Answer from the drawing. Dimensions are ordinates in mm from the lowest x, y and z of the part. Round coordinates to 2 decimals unless told otherwise and drop trailing zeros. Order: outer loops, then holes, each group sorted by start corner. A loop starts at its lowest first (then second) coordinate and runs counter-clockwise, first axis right, second up. Notation, with made-up numbers: (12.25, 57) -> (69.25, 57) arc R27 cw to (69.25, 84) -> close; hole circle Ø11 at (56, 51.25). An arc over 180 degrees is marked (long way). Use a Markdown table: item, result. Add a question column.
1. Section A-A, the plane y = 2.5 is taken. Give the vertices of the cut face in (x, z) (1 decimal).
2. Consider L1, parallel to X at y = 5, z = 6.5 (1 decimal); L2, parallel to X at y = 4.5, z = 4.75 (1 decimal); L3, parallel to Z at x = 18, y = 5 (1 decimal). Determine where each line is inside the solid, lowest interval first. Write a range as [from, to].
3. Section B-B, the plane x = 7.5 is taken. Give the vertices of the cut face in (y, z) (1 decimal).
4. Given pin 1 (6 mm diameter, centred on x = 36.5, z = 4, fed in from +Y); pin 2 (1.5 mm diameter, centred on y = 6, z = 8, fed in from -X); pin 3 (1.5 mm diameter, centred on x = 9.5, z = 10, fed in from -Y); pin 4 (1 mm diameter, centred on y = 3.5, z = 10, fed in from +X), each flat-ended and moving along its own axis, determine where each tip first touches the part or whether it passes through.
5. Section C-C, the plane z = 8.75 is taken. Give the vertices of the cut face in (x, y) (1 decimal), then the cut area to 3 significant figures.
6. The mould has two halves that part along Y. Classify the marked faces 1, 2 and 3: +Y half, -Y half, draft (parallel to the pull), parting line (faces both ways), or undercut.
7. Section D-D, the plane x = 29.5 is taken. Give the vertices of the cut face in (y, z).
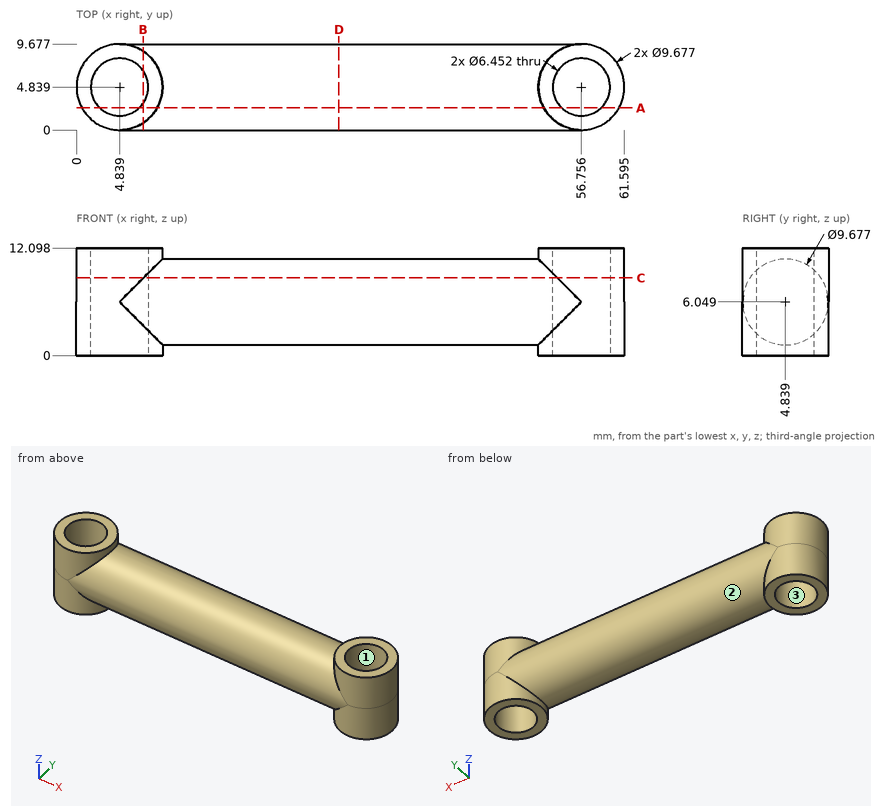
Verdict:
| question | item | result |
|---|---|---|
| 1 | outline | (0.6, 0) -> (2.6, 0) -> (2.6, 12.1) -> (0.6, 12.1) -> close; (7.1, 0) -> (9.1, 0) -> (9.1, 1.8) -> (52.5, 1.8) -> (52.5, 0) -> (54.5, 0) -> (54.5, 12.1) -> (52.5, 12.1) -> (52.5, 10.3) -> (9.1, 10.3) -> (9.1, 12.1) -> (7.1, 12.1) -> close; (59, 0) -> (61, 0) -> (61, 12.1) -> (59, 12.1) -> close |
| 2 | L1 | x = [0, 1.6], [8.1, 53.5], [60, 61.6] |
| 2 | L2 | x = [0, 1.6], [8, 53.5], [60, 61.6] |
| 2 | L3 | z = [1.2, 10.9] |
| 3 | outline | (0.8, 0) -> (3, 0) -> (3, 12.1) -> (0.8, 12.1) -> (0.8, 8.7) arc R4.8 ccw to (0.8, 3.4) -> close; (6.7, 0) -> (8.9, 0) -> (8.9, 3.4) arc R4.8 ccw to (8.9, 8.7) -> (8.9, 12.1) -> (6.7, 12.1) -> close |
| 4 | pin 1 | stops at y = 9.68 |
| 4 | pin 2 | stops at x = 0.02 |
| 4 | pin 3 | stops at y = 1.21 |
| 4 | pin 4 | stops at x = 61.52 |
| 5 | outline | (7.5, 0.8) -> (54.1, 0.8) arc R4.8 ccw (long way) to (54.1, 8.9) -> (7.5, 8.9) arc R4.8 ccw (long way) to start; hole circle Ø6.5 at (4.8, 4.8); hole circle Ø6.5 at (56.8, 4.8) |
| 5 | area | 431 mm2 |
| 6 | face 1 | undercut |
| 6 | face 2 | parting line |
| 6 | face 3 | undercut |
| 7 | outline | circle Ø9.68 at (4.84, 6.05) |
